Could you check a few things on this model? Use its own coordinates, in mm. A direction names the side the tool comes from. Coordinates: 2 decimals unless noted, no trailing zeros. Order: outer loops, then holes, each group sorted by start corner. A loop starts at its lowest first (then second) coordinate and runs counter-clockwise, first axis right, second up. Notation, with made-up numbers: (-37, -26) -> (12, -26) arc R19 ccw to (12, -7) -> close; hole circle Ø10 at (47, 38.25). An arc over 180 degrees is marked (long way). Put each result on its own line as item: value. Start each with the question number.
Q1. If we section it at A-A (y = 0): Please give me the cut outline in (x, z) (3 decimals), and give its area (3 significant figures).
Q2. We'd pull the mould along X, two halves only. Please class faces 4 (the face through (54.901, 7.776, 1.568)), 5 (the face through (-5, 0, 2)), 6 (the face through (52.123, 6.643, 1.568)): +X half, -X half, draft (parallel to the pull), parting line (faces both ways), or undercut.
Q3. Please list where these lines run through material, in increasing order: line 1 along X through (y, z) = (1.75, 1.7); line 2 along X through (y, z) = (-1, 1.6); line 3 along Y through (x, z) = (0, 0.8) (3 decimals).
Q4. If we section it at D-D (x = 41.5): Please give me the cut outline in (y, z).
Q5. For faces 1 (the face through (11, -5, 2)), 2 (the face through (43.138, 5.598, 1.568)), 3 (the face through (10, 5, 2)), which set-ups out of +Z, -Z, +X, -X, +Y, -Y let a thin tool reach every point of the face, with its end or its side?
Q6. If we section it at C-C (x = 17.5): Please give me the cut outline in (y, z).
Q7. Will these pins go through, and if not, where does the flat tip stop? pin 1 (4 mm diameter, centred on x = 38, y = 9, fed in from -Z); pin 2 (1 mm diameter, centred on y = 3.5, z = 1.5, fed in from +X).
Q8. If we section it at B-B (z = 2.6): Count the separate pieces of the cut face and the enclosed holes in it, and give its area (3 significant figures).
from build123d import *

# Parameters (mm, degrees)
SKETCH1_R           = 2.395
BOSS_EXTRUDE1_DEPTH = 3.18
FILLET1_R           = 1


with BuildPart() as part:
    # Sketch1 → Boss-Extrude1 (new body)
    # profile 1 of 2: a face of its own
    with BuildSketch(Plane.XY):
        with BuildLine():
            Line((46.303280967, 15.837507263), (19.944251464, 5))
            Line((19.944251464, 5), (22, 5))
            ThreePointArc((22, 5), (24.987746861, 4.009160597), (26.791342796, 1.429347478))
            Line((26.791342796, 1.429347478), (39.978778977, 6.851358003))
            Line((39.978778977, 6.851358003), (45.999791823, 4.461390287))
            Line((45.999791823, 4.461390287), (47.164236001, 4.258980416))
            Line((47.164236001, 4.258980416), (47.849548279, 5.221917112))
            Line((47.849548279, 5.221917112), (49.013992457, 5.019507241))
            Line((49.013992457, 5.019507241), (49.699304735, 5.982443937))
            Line((49.699304735, 5.982443937), (50.863748914, 5.780034066))
            Line((50.863748914, 5.780034066), (51.549061192, 6.742970763))
            Line((51.549061192, 6.742970763), (52.71350537, 6.540560892))
            Line((52.71350537, 6.540560892), (53.398817648, 7.503497588))
            Line((53.398817648, 7.503497588), (54.563261826, 7.301087717))
            Line((54.563261826, 7.301087717), (55.248574104, 8.264024414))
            Line((55.248574104, 8.264024414), (55.347176821, 8.304564892))
            Line((55.347176821, 8.304564892), (53.635991464, 12.466516919))
            Line((53.635991464, 12.466516919), (46.303280967, 15.837507263))
        make_face()
    # profile 2 of 2: a face of its own
    with BuildSketch(Plane.XY):
        with BuildLine():
            ThreePointArc((22, -5), (27, 0), (22, 5))
            Line((22, 5), (0, 5))
            ThreePointArc((0, 5), (-5, 0), (0, -5))
            Line((0, -5), (22, -5))
        make_face()
        with Locations(Location((22, 0, 0), (0, 0, 180))):
            Circle(SKETCH1_R, mode=Mode.SUBTRACT)
        with Locations(Location((0, 0, 0), (0, 0, 180))):
            Circle(SKETCH1_R, mode=Mode.SUBTRACT)
    extrude(amount=BOSS_EXTRUDE1_DEPTH)

    # Fillet1
    # the kernel refuses this fillet: 1 mm, written as the material it adds along each edge
    with BuildSketch(Plane(origin=(39.978778977, 6.851358003, 0), x_dir=(-0.9248782281665482, -0.3802634127332084, 0), z_dir=(0, 0, 1))) as fillet1_piece_1:
        with BuildLine():
            CenterArc((FILLET1_R * 0.404026225835, FILLET1_R), FILLET1_R, 226, 44)
            Line((-FILLET1_R * 0.290632144624, FILLET1_R * 0.280660199661), (0, 0))
            Line((0, 0), (FILLET1_R * 0.404026225835, 0))
        make_face()
    extrude(amount=3.18)
    with BuildSketch(Plane(origin=(26.791342796, 1.429347478, 0), x_dir=(0.9248782281665486, 0.38026341273320724, 0), z_dir=(0, 0, 1))) as fillet1_piece_2:
        with BuildLine():
            CenterArc((0.834537834, -1), FILLET1_R, 90, 75.522487814)
            ThreePointArc((-0.133708003, -0.75), (-0.052548991, -0.377550259), (0, 0))
            Line((0, 0), (0.834537834, 0))
        make_face()
    extrude(amount=3.18)
    with BuildSketch(Plane(origin=(19.944251464, 5, 0), x_dir=(0.9248782281665495, 0.3802634127332051, 0), z_dir=(0, 0, 1))) as fillet1_piece_3:
        with BuildLine():
            CenterArc((FILLET1_R * 0.197551931945, FILLET1_R), FILLET1_R, 247.65, 22.35)
            Line((-FILLET1_R * 0.182711480788, FILLET1_R * 0.0751217718334), (0, 0))
            Line((0, 0), (FILLET1_R * 0.197551931945, 0))
        make_face()
    extrude(amount=3.18)
    # the kernel refuses this fillet: 1 mm, written as the material it takes off along each edge
    with BuildSketch(Plane(origin=(46.303280967, 15.837507263, -1.088047115), x_dir=(-0.9248782281665417, -0.38026341273322406, 0), z_dir=(0, 0, 1))) as fillet1_2_piece_1:
        with BuildLine():
            CenterArc((FILLET1_R * 0.43521884585, FILLET1_R), FILLET1_R, 222.960833652, 47.039166348)
            Line((-FILLET1_R * 0.296600886481, FILLET1_R * 0.318501739275), (0, 0))
            Line((0, 0), (FILLET1_R * 0.43521884585, 0))
        make_face()
    extrude(amount=5.356094229, mode=Mode.SUBTRACT)
    with BuildSketch(Plane(origin=(53.635991464, 12.466516919, -0.983789259), x_dir=(-0.9085871727996149, 0.41769528298031194, 0), z_dir=(0, 0, 1))) as fillet1_2_piece_2:
        with BuildLine():
            CenterArc((FILLET1_R * 0.393515703744, FILLET1_R), FILLET1_R, 227.039166348, 42.960833652)
            Line((-FILLET1_R * 0.287982556982, FILLET1_R * 0.268180267669), (0, 0))
            Line((0, 0), (FILLET1_R * 0.393515703744, 0))
        make_face()
    extrude(amount=5.147578519, mode=Mode.SUBTRACT)
    with BuildSketch(Plane(origin=(55.347176821, 8.304564892, -1.123212767), x_dir=(-0.9248782281666527, -0.38026341273295444, 0), z_dir=(0, 0, 1))) as fillet1_2_piece_3:
        with BuildLine():
            CenterArc((1, -0.449285107), FILLET1_R, 153.302173601, 26.697826399)
            Line((0, -0.449285107), (0, 0))
            Line((0, 0), (0.106611567, 0))
        make_face()
    extrude(amount=5.426425535, mode=Mode.SUBTRACT)


solid = part.part
The answers:
1. outline: (-5, 0) -> (-2.395, 0) -> (-2.395, 3.18) -> (-5, 3.18) -> close; (2.395, 0) -> (19.605, 0) -> (19.605, 3.18) -> (2.395, 3.18) -> close; (24.395, 0) -> (27, 0) -> (27, 3.18) -> (24.395, 3.18) -> close
1. area: 71.3 mm^2
2. face 4: +X half
2. face 5: -X half
2. face 6: undercut
3. line 1: -4.68 to -1.64, 1.64 to 20.36, 23.64 to 27.57
3. line 2: -4.9 to -2.18, 2.18 to 19.82, 24.18 to 26.9
3. line 3: -5 to -2.395, 2.395 to 5
4. outline: (6.25, 0) -> (13.86, 0) -> (13.86, 3.18) -> (6.25, 3.18) -> close
5. face 1: +Z, -Z, +X, -X, -Y
5. face 2: +Z, -Z, -Y
5. face 3: +Z, -Z, -X, +Y
6. outline: (-5, 0) -> (5, 0) -> (5, 3.18) -> (-5, 3.18) -> close
7. pin 1: z = 0
7. pin 2: x = 33.04
8. separate pieces: 1
8. enclosed holes: 2
8. area: 484 mm^2
